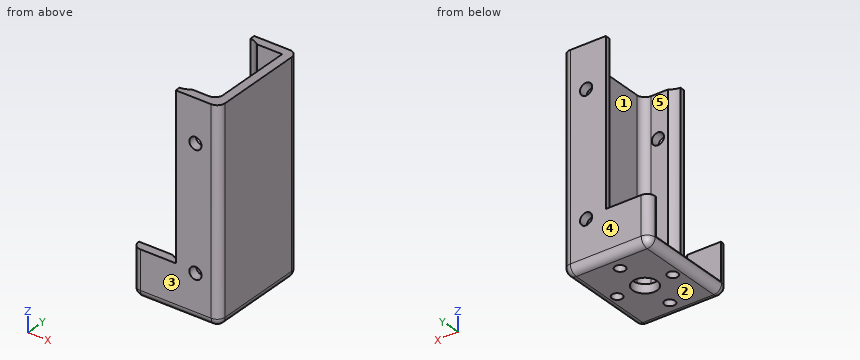
```python
from build123d import *

# Parameters (mm, degrees)
F0_W     = 19.92
F0_H     = 24.92
F0_R     = 1.5
F0_R_2   = 3.5
F0_W_2   = 2.54
F1_DEPTH = 2.54
F2_DEPTH = 60
F3_R     = 1.7526
F4_DEPTH = 34.544
F5_R     = 2.286
F7_DEPTH = 61.8236
F8_W     = 10.214
F8_H     = 46.6414740682
F9_DEPTH = 44.958


with BuildPart() as f1:
    # F0 (on Top) → F1 (new body)
    with BuildSketch(Plane.XY):
        Polygon((12.5, -15), (12.5, 15), (-12.5, 15), (-12.5, 12.46), (-9.96, 12.46), (9.96, 12.46), (9.96, -12.46), (-9.96, -12.46), (-12.5, -12.46), (-12.5, -15), align=None)
        Rectangle(F0_W, F0_H)
        with Locations((0, -9.5)):
            Circle(F0_R, mode=Mode.SUBTRACT)
        with Locations((-8, 0)):
            Circle(F0_R, mode=Mode.SUBTRACT)
        Circle(F0_R_2, mode=Mode.SUBTRACT)
        with Locations((8, 0)):
            Circle(F0_R, mode=Mode.SUBTRACT)
        with Locations((0, 9.5)):
            Circle(F0_R, mode=Mode.SUBTRACT)
        with Locations((-11.23, 0)):
            Rectangle(F0_W_2, F0_H)
    extrude(amount=F1_DEPTH)

    # F0 (on Top) → F2 (join)
    with BuildSketch(Plane.XY):
        Polygon((12.5, -15), (12.5, 15), (-12.5, 15), (-12.5, 12.46), (-9.96, 12.46), (9.96, 12.46), (9.96, -12.46), (-9.96, -12.46), (-12.5, -12.46), (-12.5, -15), align=None)
    extrude(amount=F2_DEPTH)

    # F3 (on face) → F4 (cut)
    with BuildSketch(Plane.XZ.offset(15)):
        with Locations((5.6674, 12.7526)):
            Circle(F3_R)
        with Locations((5.6674, 47.7526)):
            Circle(F3_R)
    extrude(amount=-F4_DEPTH, mode=Mode.SUBTRACT)

    # F5
    f5_edges = [f1.edges().sort_by_distance(p)[0] for p in [
        (12.5, 0, 0),
        (0, -15, 0),
        (-12.5, 0, 0),
        (0, 15, 0),
        (-12.5, -15, 30),
        (12.5, -15, 30),
        (12.5, 15, 30),
        (-12.5, 15, 30),
        (9.96, -12.46, 31.27),
    ]]
    fillet(f5_edges, radius=F5_R)

    # F6 (on face) → F7 (cut)
    with BuildSketch(Plane.XY.offset(2.54)):
        with BuildLine():
            Line((-2.6904274753, 12.46), (2.6904274753, 12.46))
            ThreePointArc((2.6904274753, 12.46), (0, 13.5), (-2.6904274753, 12.46))
        make_face()
        with BuildLine():
            Line((2.6904274753, -12.46), (-2.6904274753, -12.46))
            ThreePointArc((-2.6904274753, -12.46), (0, -13.5), (2.6904274753, -12.46))
        make_face()
    extrude(amount=F7_DEPTH, mode=Mode.SUBTRACT)

    # F8 (on face) → F9 (cut)
    with BuildSketch(Plane.XZ.offset(15)):
        Polygon((0, 64.0577673912), (-17.1696953475, 64.0577673912), (-17.1696953475, 13.3585259318), (-10.214, 13.3585259318), (-10.214, 60), (0, 60), align=None)
        with Locations((-5.107, 36.6792629659)):
            Rectangle(F8_W, F8_H)
    extrude(amount=-F9_DEPTH, mode=Mode.SUBTRACT)


solid = f1.part
```
Can you work these out from the model? Positions are in its coordinate system, mm. Face numbers are marked on the shaded views. A direction names the side the tool comes from. Give positions to 0.01 mm unless a question says otherwise; leave off trailing zeros. Order: outer loops, then holes, each group sorted by start corner. A loop starts at its lowest first (then second) coordinate and runs counter-clockwise, first axis right, second up. Notation, with made-up numbers: M 30,25 L 54,25 A28 cw 54,49 Z; hole C 81.5,54.5 d10. An arc over 180 degrees is marked long. Write item = value, one per line. Start each with the question number.
Q1. Will these pins go through, and if not, where does the flat tip stop? pin 1 Ø12 at (x, y) = (-0.5, 1.5) entering from +Z; pin 2 Ø18 at (y, z) = (5.5, 42) entering from -X; pin 3 Ø3 at (y, z) = (8, 45) entering from -X.
Q2. Suppose I cut it at C-C (y = 0). Write out the boundary of the cut face in (x, z), plus the area to 3 significant figures.
Q3. Suppose I cut it at D-D (z = 20). Write out the boundary of the cut face in (x, y).
Q4. For the marked faces 4 and 5, which set-ups out of +Z, -Z, +X, -X, +Y, -Y let a thin tool reach every point of the face, with its end or its side?
Q5. We'd pull the mould along Y, two halves only. Please class the marked faces 1, 2 and 3: pulls with the +Y half, pulls with the -Y half, needs draft (parallel to the pull), parting line crosses it, or undercut.
Q6. Suppose I cut it at B-B (y = -9.5). Write out the boundary of the cut face in (x, z).
Q7. I need wall thicknesses on probe 1 along Y at (x, z) = (7.5, 24); probe 2 along Z at (x, y) = (-3.25, 6.25); probe 3 along X at (y, z) = (3, 57.5). Which ranges of each line are inside material? Lowest first, please. Write a range as [from, to].
Q8. Suppose I cut it at A-A (x = -8). Write out the boundary of the cut face in (y, z).
Check result:
q1.pin_1 = 2.54
q1.pin_2 = 0
q1.pin_3 = 9.96
q2.outline = M -12.5,2.29 A2.29 ccw -10.21,0 L -9.5,0 L -9.5,2.54 L -12.5,2.54 Z; M -6.5,0 L -3.5,0 L -3.5,2.54 L -6.5,2.54 Z; M 3.5,0 L 6.5,0 L 6.5,2.54 L 3.5,2.54 Z; M 9.5,0 L 10.21,0 A2.29 ccw 12.5,2.29 L 12.5,60 L 9.96,60 L 9.96,2.54 L 9.5,2.54 Z
q2.area = 174 mm2
q3.outline = M 0,-15 L 10.21,-15 A2.29 ccw 12.5,-12.71 L 12.5,12.71 A2.29 ccw 10.21,15 L 0,15 L 0,13.5 A4 cw 2.69,12.46 L 9.96,12.46 L 9.96,-10.17 A2.29 cw 7.67,-12.46 L 2.69,-12.46 A4 cw 0,-13.5 Z
q4.face_4 = +Z, -Z, +X, -X, +Y
q4.face_5 = +Z, -X
q5.face_1 = undercut
q5.face_2 = needs draft
q5.face_3 = pulls with the -Y half
q6.outline = M -12.5,2.29 A2.29 ccw -10.21,0 L -1.5,0 L -1.5,2.54 L -12.5,2.54 Z; M 1.5,0 L 10.21,0 A2.29 ccw 12.5,2.29 L 12.5,60 L 9.96,60 L 9.96,2.54 L 1.5,2.54 Z
q7.probe_1 = [-15, -12.46], [12.46, 15]
q7.probe_2 = [0, 2.54]
q7.probe_3 = [9.96, 12.5]
q8.outline = M -15,2.29 A2.29 ccw -12.71,0 L -1.5,0 L -1.5,2.54 L -12.46,2.54 L -12.46,13.36 L -15,13.36 Z; M 1.5,0 L 12.71,0 A2.29 ccw 15,2.29 L 15,13.36 L 12.46,13.36 L 12.46,2.54 L 1.5,2.54 Z
